Autodesk Inventor part; units mm, degrees
ref_plane "YZ Plane" through (0, 0, 0) normal (1, 0, 0) x (0, 1, 0)
ref_plane "XZ Plane" through (0, 0, 0) normal (0, 1, 0) x (-1, 0, 0)
ref_plane "XY Plane" through (0, 0, 0) normal (0, 0, 1) x (1, 0, 0)
sketch "Эскиз1" plane through (0, 0, 0) normal (0, 0, 1) x (1, 0, 0)
  line L0 (22, -11.5) -> (-22, -11.5)
  line L1 (-22, -11.5) -> (-22, 11.5)
  line L2 (-22, 11.5) -> (22, 11.5)
  line L3 (22, 11.5) -> (22, -11.5)
  line L4 (22, -11.5) -> (-22, 11.5) construction
  line L5 (-22, -11.5) -> (22, 11.5) construction
  line L6 (20, -10.4545) -> (-20, 10.4545) construction
  line L7 (-20, -10.4545) -> (20, 10.4545) construction
  line L8 (21, -10.5) -> (-21, -10.5)
  line L9 (-21, -10.5) -> (-21, 10.5)
  line L10 (-21, 10.5) -> (21, 10.5)
  line L11 (21, 10.5) -> (21, -10.5)
  line L12 (21, -10.5) -> (-21, 10.5) construction
  line L13 (-21, -10.5) -> (21, 10.5) construction
  point P0 (0, 0)
  dimension "d0" = 23
  dimension "d1" = 44
  dimension "d3" = 1
  dimension "d4" = 1
  dimension "d5" = 1
extrude "Выдавливание1" add sketch "Эскиз1" along normal blind 20
sketch "Эскиз3" plane through (0, 0, 20) normal (0, 0, 1) x (1, 0, 0)
  line L0 (22, 11.5) -> (-22, 11.5)
  line L1 (-22, -11.5) -> (22, -11.5)
  line L2 (-22, 11.5) -> (22, 11.5)
  line L3 (22, 11.5) -> (22, -11.5)
  line L4 (22, -11.5) -> (-22, -11.5)
  line L5 (-22, -11.5) -> (-22, 11.5)
  point P0 (0, 0)
extrude "Выдавливание2" add sketch "Эскиз3" along normal blind 1
sketch "Эскиз4" plane through (0, 0, 0) normal (0, 0, -1) x (-1, 0, 0)
  line L0 (25, -6.3038) -> (25, 6.3038)
  line L1 (-22, 11.5) -> (22, 11.5)
  line L2 (25, 6.3038) -> (22, 11.5)
  line L3 (22, -11.5) -> (-22, -11.5)
  line L4 (22, 11.5) -> (22, -11.5)
  line L5 (22, -11.5) -> (25, -6.3038)
  line L6 (-22, -11.5) -> (-22, 11.5)
  line L7 (-22, -11.5) -> (-22, 11.5)
  line L8 (-22, 11.5) -> (-25, 6.3038)
  line L9 (-25, 6.3038) -> (-25, -6.3038)
  line L10 (-25, -6.3038) -> (-22, -11.5)
  point P0 (0, 0)
  dimension "d10" = 3
  dimension "d11" = 3
  dimension "d12" = 30
  dimension "d13" = 30
  dimension "d14" = 30
  dimension "d15" = 30
extrude "Выдавливание3" add sketch "Эскиз4" against normal blind 1 contours L5 L4 L2 L0 | L10 L9 L8 L6
sketch "Эскиз5" plane through (0, 0, 0) normal (0, 0, -1) x (-1, 0, 0)
  line L0 (-21, 10.5) -> (-21, -10.5)
  line L1 (-21, -10.5) -> (21, -10.5)
  line L2 (21, -10.5) -> (21, 10.5)
  line L3 (21, 10.5) -> (-21, 10.5)
  line L4 (22, -11.5) -> (-22, -11.5)
  line L5 (-22, -11.5) -> (-22, 11.5)
  line L6 (-22, 11.5) -> (22, 11.5)
  line L7 (22, 11.5) -> (22, -11.5)
  point P0 (0, 0)
extrude "Выдавливание4" add sketch "Эскиз5" along normal blind 2
properties part number "кейсик"
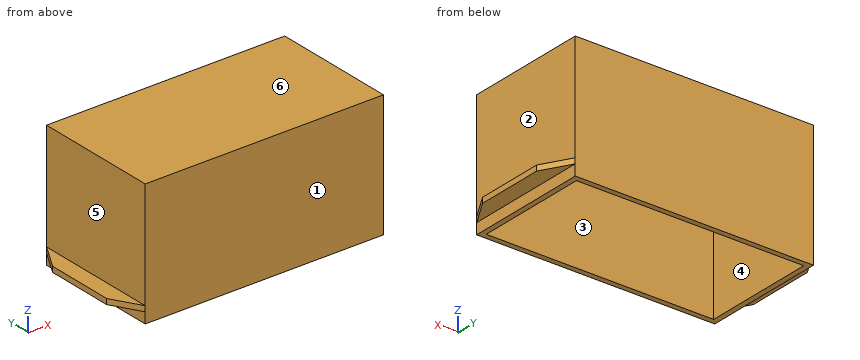
Can you work these out from the model? Positions are in its coordinate system, mm. Face numbers are marked on the shaded views. A direction names the side the tool comes from. Give positions to 0.01 mm unless a question says otherwise; leave off trailing zeros. Order: outer loops, then holes, each group sorted by start corner. A loop starts at its lowest first (then second) coordinate and runs counter-clockwise, first axis right, second up. Notation, with made-up numbers: (83, 17) - (88, 17) arc R22 ccw to (88, 35) - close; hole circle Ø2 at (53, 82). An arc over 180 degrees is marked (long way). Use a Markdown table: item, result. Add a question column.
Q1. If we mould it in two halves opening along X, with no side actions, what happens to the marked faces 3, 4, 5 and 6? For each: released by +X, released by -X, zero draft, split by the parting line, or undercut.
Q2. If we section it at A-A on z = 5: Write out the boundary of the cut face in (x, y).
Q3. I'm going to push flat-ended pins straight in: pin 1 (1.5 mm diameter, centred on x = -23.5, y = -2.5, fed in from +Z); pin 2 (2 mm diameter, centred on x = 19.5, y = -6, fed in from -Z); pin 3 (0.6 mm diameter, centred on y = 2.5, z = -1, fed in from -X). Where does each tip first touch, or does it pass through?
Q4. If we section it at C-C on y = 3: Write out the boundary of the cut face in (x, z).
Q5. On a 3-axis mill with a long thin cutter (end or side, diameter ignored), from which of +Z, -Z, +X, -X, +Y, -Y can I reach the whole of each face in a straight line? I mean the marked faces 1 and 2. Say none if no direction works.
Q6. Please list where these lines run through material, in increasing order: line 1 along X through (y, z) = (-6.75, 9.5); line 2 along Y through (x, z) = (0.5, 2.25); line 3 along Z through (x, y) = (-1, -7).
Q7. If we section it at B-B on x = 11: Write out the boundary of the cut face in (y, z), plus the area to 3 significant figures.
Answers follow:
| question | item | result |
|---|---|---|
| 1 | face 3 | undercut |
| 1 | face 4 | undercut |
| 1 | face 5 | released by -X |
| 1 | face 6 | zero draft |
| 2 | outline | (-22, -11.5) - (22, -11.5) - (22, 11.5) - (-22, 11.5) - close; hole (-21, -10.5) - (21, -10.5) - (21, 10.5) - (-21, 10.5) - close |
| 3 | pin 1 | stops at z = 1 |
| 3 | pin 2 | stops at z = 20 |
| 3 | pin 3 | stops at x = -22 |
| 4 | outline | (-25, 0) - (-22, 0) - (-22, -2) - (-21, -2) - (-21, 20) - (21, 20) - (21, -2) - (22, -2) - (22, 0) - (25, 0) - (25, 1) - (22, 1) - (22, 21) - (-22, 21) - (-22, 1) - (-25, 1) - close |
| 5 | face 1 | +Z, -Z, +X, -X, -Y |
| 5 | face 2 | +Z, +X, +Y, -Y |
| 6 | line 1 | x = -22 to -21, 21 to 22 |
| 6 | line 2 | y = -11.5 to -10.5, 10.5 to 11.5 |
| 6 | line 3 | z = 20 to 21 |
| 7 | outline | (-11.5, -2) - (-10.5, -2) - (-10.5, 20) - (10.5, 20) - (10.5, -2) - (11.5, -2) - (11.5, 21) - (-11.5, 21) - close |
| 7 | area | 67.0 mm^2 |
